The model under review builds one solid part; all positions refer to its coordinate system, in mm. A direction names the side the tool comes from. Coordinates: 2 decimals unless noted, no trailing zeros. Write each loop counter-clockwise with the first axis right and the second up, starting at its lowest first coordinate (ties: lowest second). Pieces come first, ordered by that corner, then holes. Notation, with made-up numbers: (56.25, 10) - (66.25, 10) arc R11 ccw to (66.25, 18) - close; hole circle Ø9 at (-1.5, 64.25). An arc over 180 degrees is marked (long way). Return JSON: item names as keys, results as strings. Group by question number.
(1) We need section A-A on x = 88. State the section outline as (y, z) points, then the cut area to 3 significant figures.
(2) We need section C-C on z = -9.25. State the section outline as (x, y) points.
(3) Draft analysis for pull direction Z (two halves, no side actions). For faces 1 (the face through (73.533, 3.155, -8.355)), 2 (the face through (85.6, 3.16, -5.36)), 3 (the face through (93.3, 0, -7.3)), 4 (the face through (89, 3, -15.883)), state which applies: released by +Z, released by -Z, zero draft, split by the parting line, or undercut.
(4) We need section B-B on y = 0.5. State the section outline as (x, z) points (1 decimal).
(5) To check wall thickness, follow L1, parallel to X at y = 6, z = -7.5; L2, parallel to Z at x = 87.5, y = 1; L3, parallel to X at y = 2, z = -6.25. State the ranges of each line that lie inside material, in increasing order. Write a range as from..to.
(6) Tool access review of faces 5 (the face through (104.715, 3.155, -13.665)), 6 (the face through (76, 6.3, -11)): name each direction out of +Z, -Z, +X, -X, +Y, -Y from which nothing blocks a thin tool from reaching the whole face with its end or side.
(7) We need section D-D on z = -12. State the section outline as (x, y) points, then the cut area to 3 significant figures.
```python
from build123d import *

# Parameters (mm, degrees)
SKETCH1_R           = 3.9125
SKETCH1_R_2         = 1.5
BOSS_EXTRUDE1_DEPTH = 6.4
SKETCH2_W           = 1
SKETCH2_H           = 1
CUT_EXTRUDE1_DEPTH  = 0.1


with BuildPart() as part:
    # Sketch1 → Boss-Extrude1 (new body)
    with BuildSketch(Plane(origin=(0, 0, 0), x_dir=(1, 0, 0), z_dir=(0, 1, 0))):
        Polygon((102.49610132, 15.883489834), (106.99610132, 11.383489834), (106.99610132, 2.946691354), (102.49610132, -1.553308646), (75.64610132, -1.553308646), (71.14610132, 2.946691354), (71.14610132, 11.383489834), (75.64610132, 15.883489834), align=None)
        with Locations(Location((89.07110132, 7.165090594, 0), (0, 0, 270))):
            Circle(SKETCH1_R, mode=Mode.SUBTRACT)
        with Locations(Location((74.44610132, 7.165090594, 0), (0, 0, 270))):
            Circle(SKETCH1_R_2, mode=Mode.SUBTRACT)
        with Locations(Location((103.69610132, 7.165090594, 0), (0, 0, 90))):
            Circle(SKETCH1_R_2, mode=Mode.SUBTRACT)
    extrude(amount=BOSS_EXTRUDE1_DEPTH)

    # Sketch2 → Cut-Extrude1 (cut)
    with BuildSketch(Plane(origin=(0, 6.4, 0), x_dir=(1, 0, 0), z_dir=(0, 1, 0))):
        with Locations((75.696023721, 10.665090594)):
            Rectangle(SKETCH2_W, SKETCH2_H)
    extrude(amount=-CUT_EXTRUDE1_DEPTH, mode=Mode.SUBTRACT)


solid = part.part
```
Ans:
{
 "1": {"outline": "(0, -15.88) - (6.4, -15.88) - (6.4, -10.93) - (0, -10.93) - close; (0, -3.4) - (6.4, -3.4) - (6.4, 1.55) - (0, 1.55) - close", "area": "63.4 mm²"},
 "2": {"outline": "(71.15, 0) - (85.76, 0) - (85.76, 6.4) - (71.15, 6.4) - close; (92.38, 0) - (107, 0) - (107, 6.4) - (92.38, 6.4) - close"},
 "3": {"face 1": "undercut", "face 2": "undercut", "face 3": "zero draft", "face 4": "released by -Z"},
 "4": {"outline": "(71.1, -11.4) - (75.6, -15.9) - (102.5, -15.9) - (107, -11.4) - (107, -2.9) - (102.5, 1.6) - (75.6, 1.6) - (71.1, -2.9) - close; hole circle Ø3 at (74.4, -7.2); hole circle Ø7.8 at (89.1, -7.2); hole circle Ø3 at (103.7, -7.2)"},
 "5": {"L1": "71.15..72.98, 75.91..85.17, 92.97..102.23, 105.16..107", "L2": "-15.88..-10.75, -3.58..1.55", "L3": "71.15..73.26, 75.63..85.27, 92.88..102.51, 104.88..107"},
 "6": {"face 5": "-Z, +X, +Y, -Y", "face 6": "+Y"},
 "7": {"outline": "(71.76, 0) - (106.38, 0) - (106.38, 6.4) - (71.76, 6.4) - close", "area": "222 mm²"}
}
